Check sheet for the modelled part. Datum: model origin and axes. Units: mm. Coordinates: 2 decimals unless noted, no trailing zeros. Write each loop counter-clockwise with the first axis right and the second up, starting at its lowest first coordinate (ties: lowest second). Pieces come first, ordered by that corner, then holes. Notation, with made-up numbers: M 71.5,-11.75 L 75.5,-11.75 A29 ccw 75.5,11.25 Z; hole C -23,65.5 d11. An arc over 180 degrees is marked long. Answer as CSV lines item,"result". Start each with the question number.
Q1. Sectioned sample at D-D, the plane z = 27. Record the cut outline in (x, y).
Q2. Sectioned sample at A-A, the plane z = 65. Record the cut outline in (x, y).
Q3. Thickness scan on line 1 along Z through (x, y) = (-4.7, 0); line 2 along Y through (x, z) = (-1.5, 63). Record the ranges inside material, lowest first. Write a range as from..to.
Q4. Sectioned sample at B-B, the plane x = -2.75. Record the cut outline in (y, z).
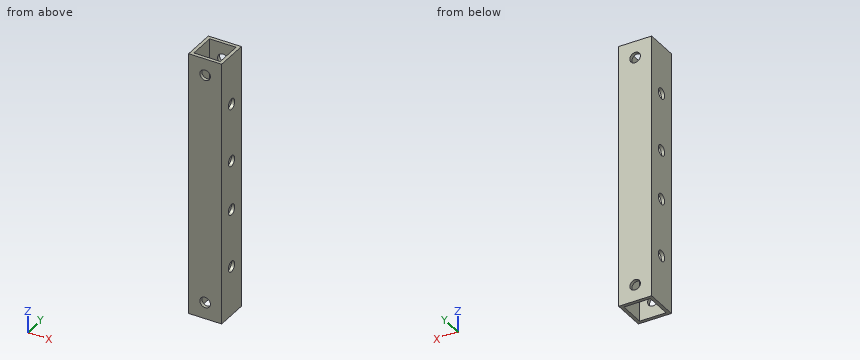
from build123d import *

# Parameters (mm, degrees)
SKETCH_1_W          = 10
SKETCH_1_H          = 10
SKETCH_1_W_2        = 8
SKETCH_1_H_2        = 8
EXTRUDE_1_DEPTH     = 80
SKETCH_2_R          = 1.6
CUT_EXTRUDE_1_DEPTH = 81.777472107
SKETCH_3_R          = 1.6
CUT_EXTRUDE_2_DEPTH = 81.777472107


with BuildPart() as part:
    # ｽｹｯﾁ1 → ﾎﾞｽ - 押し出し1 (new body)
    with BuildSketch(Plane.XY):
        Rectangle(SKETCH_1_W, SKETCH_1_H)
        Rectangle(SKETCH_1_W_2, SKETCH_1_H_2, mode=Mode.SUBTRACT)
    extrude(amount=EXTRUDE_1_DEPTH)

    # ｽｹｯﾁ2 → ｶｯﾄ - 押し出し1 (cut, through all)
    with BuildSketch(Plane.ZY.offset(5)):
        with Locations(Location((15, 0, 0), (0, 0, 270))):
            Circle(SKETCH_2_R)
        with Locations(Location((65, 0, 0), (0, 0, 270))):
            Circle(SKETCH_2_R)
        with Locations(Location((32.5, 0, 0), (0, 0, 270))):
            Circle(SKETCH_2_R)
        with Locations(Location((47.5, 0, 0), (0, 0, 270))):
            Circle(SKETCH_2_R)
    extrude(amount=-CUT_EXTRUDE_1_DEPTH, mode=Mode.SUBTRACT)

    # ｽｹｯﾁ3 → ｶｯﾄ - 押し出し2 (cut, through all)
    with BuildSketch(Plane(origin=(0, 5, 0), x_dir=(1, 0, 0), z_dir=(0, 1, 0))):
        with Locations(Location((0, -5, 0), (0, 0, 270))):
            Circle(SKETCH_3_R)
        with Locations(Location((0, -75, 0), (0, 0, 270))):
            Circle(SKETCH_3_R)
    extrude(amount=-CUT_EXTRUDE_2_DEPTH, mode=Mode.SUBTRACT)


solid = part.part
Output:
1,outline,"M -5,-5 L 5,-5 L 5,5 L -5,5 Z; hole M -4,-4 L 4,-4 L 4,4 L -4,4 Z"
2,outline,"M -5,-5 L 5,-5 L 5,-1.6 L 4,-1.6 L 4,-4 L -4,-4 L -4,-1.6 L -5,-1.6 Z; M -5,1.6 L -4,1.6 L -4,4 L 4,4 L 4,1.6 L 5,1.6 L 5,5 L -5,5 Z"
3,line 1,"z = 0..13.4, 16.6..30.9, 34.1..45.9, 49.1..63.4, 66.6..80"
3,line 2,"y = -5..-4, 4..5"
4,outline,"M -5,0 L -4,0 L -4,80 L -5,80 Z; M 4,0 L 5,0 L 5,80 L 4,80 Z"
